For this review, take the finished solid that the model builds, in its own axes (mm). A direction names the side the tool comes from. Coordinates: 2 decimals unless noted, no trailing zeros. Loops run counter-clockwise (first coordinate to the right, second up) from the corner with the lowest first, then second, coordinate; pieces in that order, holes last. Notation, with made-up numbers: (70.5, 2.5) -> (115.5, 2.5) arc R29 ccw to (115.5, 28.5) -> close; hole circle Ø10 at (83.5, 59). An arc over 180 degrees is marked (long way). Use a Markdown table: item, result.
from build123d import *

# Parameters (mm, degrees)
CYLINDER030_R         = 8
CYLINDER030_DEPTH     = 4
CYLINDER056_R         = 3
CYLINDER056_DEPTH     = 20
POLARPATTERN011_COUNT = 8
CYLINDER057_R         = 3.5
CYLINDER057_DEPTH     = 24


with BuildPart() as part:
    # Cone → Cone (revolve)
    with BuildSketch(Plane.XZ):
        Polygon((0, 0), (11, 0), (8, 20), (0, 20), align=None)
    revolve(axis=Axis((0, 0, 0), (0, 0, 1)))

    # Cylinder030 → Cylinder030 (join)
    with BuildSketch(Plane.XY.offset(20)):
        Circle(CYLINDER030_R)
    extrude(amount=CYLINDER030_DEPTH)

    # Cylinder056 → Cylinder056 (cut)
    with BuildSketch(Plane(origin=(11, 0, 0), x_dir=(1, 0, 0), z_dir=(0, 0, 1))):
        Circle(CYLINDER056_R)
    cylinder056 = extrude(amount=CYLINDER056_DEPTH, mode=Mode.SUBTRACT)

    # PolarPattern011: Cylinder056 ×8 about axis
    polarpattern011_axis = Axis((0, 0, 0), (0, 0, 1))
    for i in range(1, POLARPATTERN011_COUNT):
        add(cylinder056.rotate(polarpattern011_axis, i * 360 / POLARPATTERN011_COUNT), mode=Mode.SUBTRACT)

    # Cylinder057 → Cylinder057 (cut)
    with BuildSketch(Plane.XY):
        Circle(CYLINDER057_R)
    extrude(amount=CYLINDER057_DEPTH, mode=Mode.SUBTRACT)


with BuildPart() as part_1:
    # Body017 placement: moved
    add(part.part.moved(Location((-38, 0, 0))))


solid = part_1.part
(1) For faces 1 (the face through (-38, -8, 8)), 2 (the face through (-44.349, -4.868, 21.972)), list the 3-axis set-ups (+Z, -Z, +X, -X, +Y, -Y) from which the entire face can be reached by the end or side of a thin tool; tool diameter is ignored.
Found:
| item | result |
|---|---|
| face 1 | +Z, -Z, -Y |
| face 2 | +Z |
(2) For line 1 along Y through (x, z) = (-38, 13.5); line 2 along X through (y, z) = (-3, 17.75); line 3 along X through (y, z) = (8.25, 3.5), list the stretches that pass through material, from the lowest coordinate up.
Found:
| item | result |
|---|---|
| line 1 | y = -8 to -3.5, 3.5 to 8 |
| line 2 | x = -45.78 to -39.8, -36.2 to -30.22 |
| line 3 | x = -42.82 to -39.2, -36.8 to -33.18 |
(3) For pin 1 Ø6 at (x, z) = (-34.5, 6) entering from -Y; pin 2 Ø6 at (y, z) = (6.5, 3) entering from -X; pin 3 Ø3 at (x, z) = (-43.5, 16.5) entering from -Y, all flat-tipped, find the tip position at first contact; note any pin that passes through.
Found:
| item | result |
|---|---|
| pin 1 | stops at y = -10.14 |
| pin 2 | stops at x = -48.05 |
| pin 3 | stops at y = -7.57 |
(4) Take a section at A-A on z = 21. Write out the cut boundary in (x, y), plus the area to 3 significant figures.
Found:
| item | result |
|---|---|
| outline | circle Ø16 at (-38, 0); hole circle Ø7 at (-38, 0) |
| area | 163 mm^2 |
(5) Take a section at B-B on z = 8. Write out the cut boundary in (x, y).
Found:
| item | result |
|---|---|
| outline | (-47.46, -2.57) arc R9.8 ccw to (-46.51, -4.87) arc R3 cw to (-42.87, -8.51) arc R9.8 ccw to (-40.57, -9.46) arc R3 cw to (-35.43, -9.46) arc R9.8 ccw to (-33.13, -8.51) arc R3 cw to (-29.49, -4.87) arc R9.8 ccw to (-28.54, -2.57) arc R3 cw to (-28.54, 2.57) arc R9.8 ccw to (-29.49, 4.87) arc R3 cw to (-33.13, 8.51) arc R9.8 ccw to (-35.43, 9.46) arc R3 cw to (-40.57, 9.46) arc R9.8 ccw to (-42.87, 8.51) arc R3 cw to (-46.51, 4.87) arc R9.8 ccw to (-47.46, 2.57) arc R3 cw to start; hole circle Ø7 at (-38, 0) |
